Check sheet for the drawn part. Datum: minimum x, y, z corner. Units: mm. A direction names the side the tool comes from. Round coordinates to 2 decimals unless told otherwise and drop trailing zeros. Write each loop counter-clockwise with the first axis right and the second up, starting at its lowest first coordinate (ties: lowest second). Pieces come first, ordered by that corner, then holes.
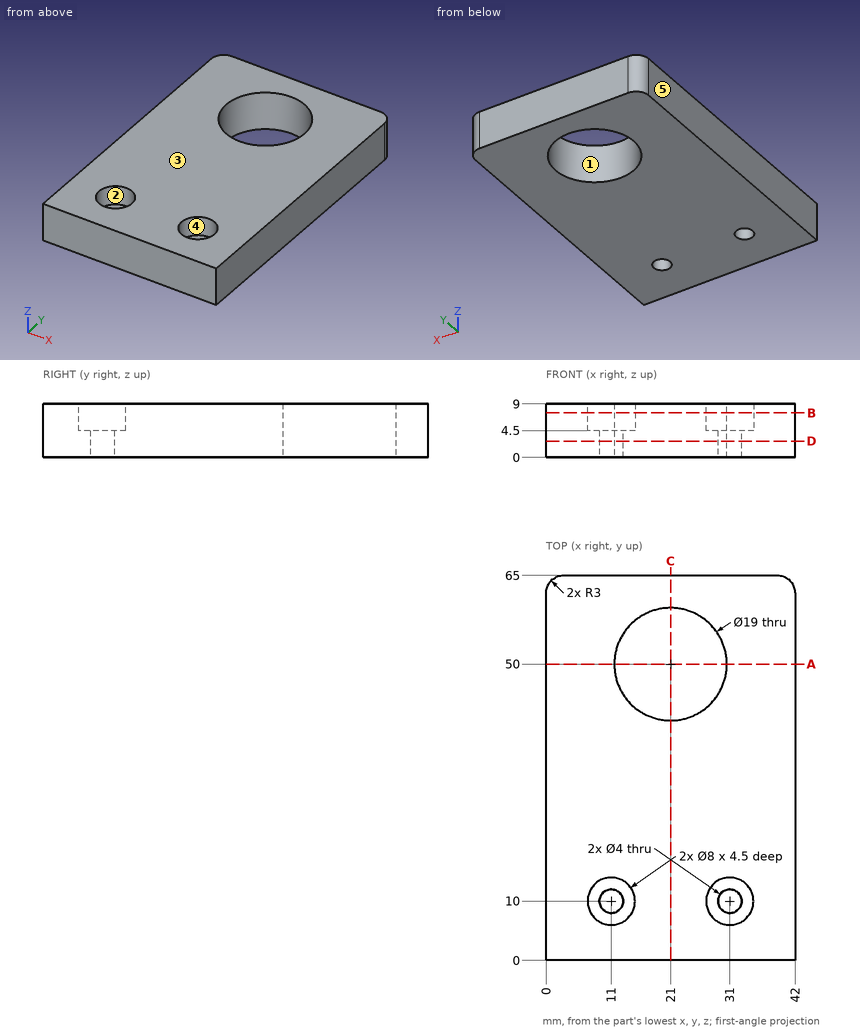
Q1. Depth check by flat-ended pin: P1, Ø1.5, axis at x = 7, y = 29, coming from the -Z side; P2, Ø4, axis at x = 12, y = 9, coming from the +Z side. Enter the tip coordinate at first touch or a pass-through.
Recorded:
P1: stops at z = 0
P2: stops at z = 4.5
Q2. Tool access check on the marked faces 1 and 2. Record the directions out of +Z, -Z, +X, -X, +Y, -Y that give a thin tool (end or side, any length) a straight path to the whole face; none if there is none.
Recorded:
face 1: +Z, -Z
face 2: +Z
Q3. Release check for a two-part mould opening along X. For the marked faces 3, 4 and 5 record: released by +X, released by -X, zero draft, split by the parting line, or undercut.
Recorded:
face 3: zero draft
face 4: undercut
face 5: released by -X
Q4. Sectioned sample at D-D (z = 2.75). Enter the section's corners in (x, y), plus the area to 3 significant figures.
Recorded:
outline: (0, 0) - (42, 0) - (42, 62) arc R3 ccw to (39, 65) - (3, 65) arc R3 ccw to (0, 62) - close; hole circle Ø4 at (11, 10); hole circle Ø19 at (21, 50); hole circle Ø4 at (31, 10)
area: 2,420 mm2
Q5. Sectioned sample at C-C (x = 21). Enter the section's corners in (y, z), plus the area to 3 significant figures.
Recorded:
outline: (0, 0) - (40.5, 0) - (40.5, 9) - (0, 9) - close; (59.5, 0) - (65, 0) - (65, 9) - (59.5, 9) - close
area: 414 mm2
Q6. Sectioned sample at B-B (z = 7.5). Enter the section's corners in (x, y), plus the area to 3 significant figures.
Recorded:
outline: (0, 0) - (42, 0) - (42, 62) arc R3 ccw to (39, 65) - (3, 65) arc R3 ccw to (0, 62) - close; hole circle Ø8 at (11, 10); hole circle Ø19 at (21, 50); hole circle Ø8 at (31, 10)
area: 2,340 mm2
Q7. Sectioned sample at A-A (y = 50). Enter the section's corners in (x, z), plus the area to 3 significant figures.
Recorded:
outline: (0, 0) - (11.5, 0) - (11.5, 9) - (0, 9) - close; (30.5, 0) - (42, 0) - (42, 9) - (30.5, 9) - close
area: 207 mm2
Q8. Material ranges on line 1 along X through (y, z) = (10, 1.05); line 2 along Y through (x, z) = (21, 4); line 3 along Y through (x, z) = (31, 1.8), recorded low to high.
Recorded:
line 1: x = 0 to 9, 13 to 29, 33 to 42
line 2: y = 0 to 40.5, 59.5 to 65
line 3: y = 0 to 8, 12 to 65
